The figure shows three views and two pictorial views of one solid part (mm, origin at its lowest corner). Answer the questions. A direction names the side the tool comes from. Coordinates: 2 decimals unless noted, no trailing zeros. Write each loop counter-clockwise with the first axis right and the second up, starting at its lowest first coordinate (ties: lowest second). Pieces come first, ordered by that corner, then holes. Notation, with made-up numbers: M -12,12 L 40,12 A25 ccw 40,48 Z; hole C 58.5,15.5 d9. An arc over 180 degrees is marked long. Use a Markdown table: item, result. Add a question column.
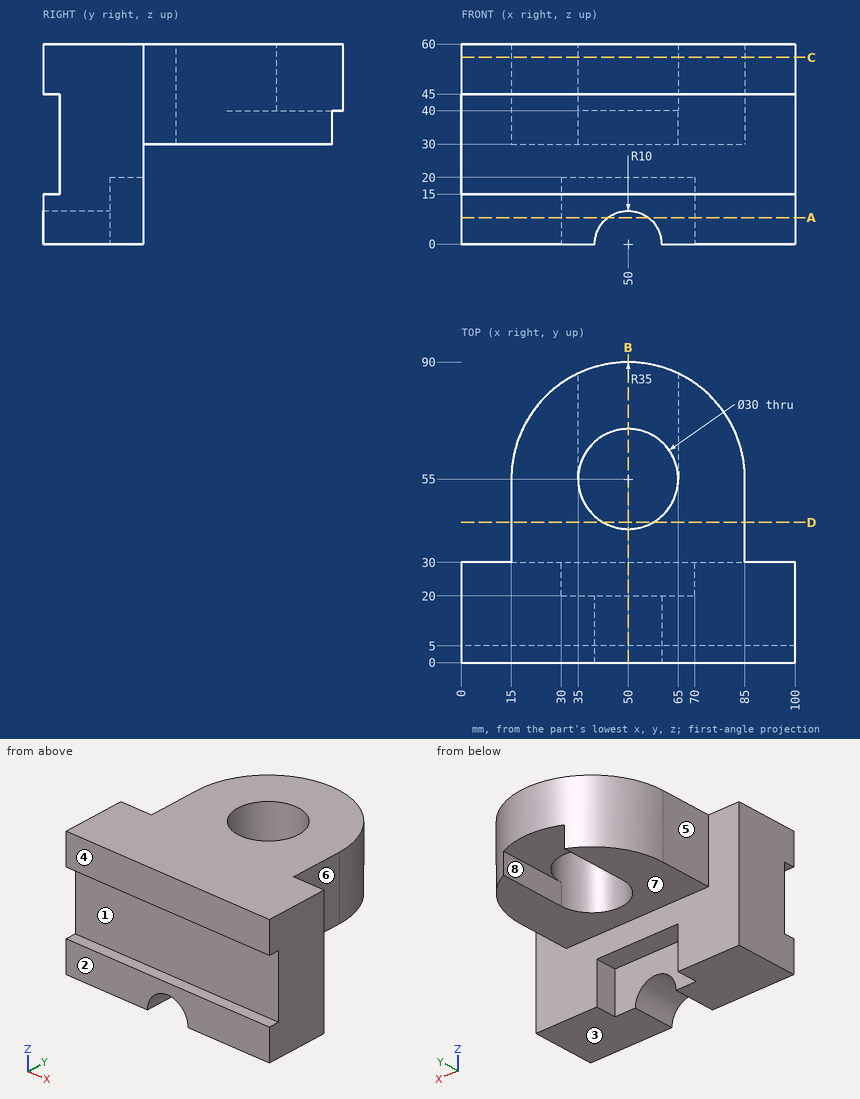
Item 1: Each of these flat-tipped pins is pushed along its axis until it touches: pin 1 (8 mm diameter, centred on y = 69, z = 34, fed in from +X); pin 2 (24 mm diameter, centred on x = 51.5, y = 68, fed in from -Z); pin 3 (12 mm diameter, centred on x = 89.5, z = 12.5, fed in from +Y). Where does it stop, or does it pass through?
Item 2: For the marked faces 4, 5, 6, 7 and 8, determine the directions among +Z, -Z, +X, -X, +Y, -Y from which every point of the face is accessible in a straight line to the end or side of a thin tool.
Item 3: Determine the mould class of the marked faces 1, 2 and 3 for opening direction Z: pulls with the +Z half, pulls with the -Z half, needs draft (parallel to the pull), parting line crosses it, or undercut.
Item 4: Find section B-B on x = 50. Give the vertices of the cut face in (y, z).
Item 5: Consider probe 1 along Y at (x, z) = (50, 50); probe 2 along X at (y, z) = (55, 38); probe 3 along Y at (x, z) = (72.5, 21.5). Determine where each line is inside the solid, lowest interval first.
Item 6: Find section C-C on z = 56. Give the vertices of the cut face in (x, y).
Item 7: Find section D-D on y = 42. Give the vertices of the cut face in (x, z).
Item 8: Find section A-A on z = 8. Give the vertices of the cut face in (x, y), then the cut area to 3 significant figures.
Geometry says:
| question | item | result |
|---|---|---|
| 1 | pin 1 | stops at x = 83.54 |
| 1 | pin 2 | stops at z = 40 |
| 1 | pin 3 | stops at y = 30 |
| 2 | face 4 | +Z, -Z, +X, -X, -Y |
| 2 | face 5 | +Z, -Z, -X, +Y |
| 2 | face 6 | +Z, -Z, +X, +Y |
| 2 | face 7 | -Z, +X, -X, +Y |
| 2 | face 8 | -Z, +Y |
| 3 | face 1 | undercut |
| 3 | face 2 | needs draft |
| 3 | face 3 | pulls with the -Z half |
| 4 | outline | M 0,10 L 20,10 L 20,20 L 30,20 L 30,30 L 40,30 L 40,60 L 0,60 L 0,45 L 5,45 L 5,15 L 0,15 Z; M 70,40 L 90,40 L 90,60 L 70,60 Z |
| 5 | probe 1 | y = 0 to 40, 70 to 90 |
| 5 | probe 2 | x = 15 to 35, 65 to 85 |
| 5 | probe 3 | y = 5 to 30 |
| 6 | outline | M 0,0 L 100,0 L 100,30 L 85,30 L 85,55 A35 ccw 15,55 L 15,30 L 0,30 Z; hole C 50,55 d30 |
| 7 | outline | M 15,30 L 42.52,30 L 42.52,60 L 15,60 Z; M 57.48,30 L 85,30 L 85,60 L 57.48,60 Z |
| 8 | outline | M 0,0 L 44,0 L 44,20 L 30,20 L 30,30 L 0,30 Z; M 56,0 L 100,0 L 100,30 L 70,30 L 70,20 L 56,20 Z |
| 8 | area | 2,360 mm2 |
